Geometry: final body of the model. Coordinates: model frame, mm. Coordinates: 2 decimals unless noted, no trailing zeros. Loops run counter-clockwise (first coordinate to the right, second up) from the corner with the lowest first, then second, coordinate; pieces in that order, holes last. Notation, with made-up numbers: (17.5, 60) -> (59.5, 60) arc R24 ccw to (59.5, 81) -> close; hole circle Ø2 at (51, -26.5). An arc over 180 degrees is marked (long way). One line per item, written item: value. Start each with the question number.
Item 1: Section query B-B on x = 0. Return loops of the section in (y, z), then the cut area to 3 significant figures.
Item 2: Section query D-D on z = 28.5. Return loops of the section in (x, y), then the cut area to 3 significant figures.
Item 3: Ray query, probe 1 along Z at (x, y) = (0, 8.85); probe 2 along Z at (x, y) = (0, 7.35); probe 3 along X at (y, z) = (9, 38). Return the intervals inside material, ascending. Write a range as from..to.
Item 4: Contact query for flat-ended pins moving along their axis: pin 1 Ø1 at (x, y) = (-5.5, 7.5) entering from -Z; pin 2 Ø1 at (x, z) = (-3, 20.5) entering from -Y; pin 3 Ø4 at (x, z) = (0, 23.6) entering from -Y; pin 4 Ø2 at (y, z) = (6, 32.5) entering from -X. Output: stop coordinate, or through.
Item 5: Mould query, pull axis Y, two halves, no side actions, for faces 1 (the cylindrical face through (0.07, 9.27, 37.53)), 2 (the flat face through (0, 7, 0)), 3 (the cylindrical face through (-3.21, 9.47, 23.27)), 4 (the flat face through (8, 0, 23)). Classes: +Y half, -Y half, draft (parallel to the pull), parting line (faces both ways), or undercut.
Item 6: Section query A-A on y = 5.25. Return loops of the section in (x, z), then the cut area to 3 significant figures.
Item 7: Section query C-C on z = 23.6. Return loops of the section in (x, y), then the cut area to 3 significant figures.
from build123d import *

# Parameters (mm, degrees)
BOSS_EXTRUDE1_DEPTH     = 47.2
CUT_EXTRUDE1_DEPTH      = 50.273116402
CUT_EXTRUDE1_DEPTH_BACK = 50.273116402
SKETCH3_R               = 1.5
CUT_EXTRUDE3_DEPTH      = 51.597430898
CUT_EXTRUDE3_DEPTH_BACK = 51.597430898
SKETCH7_R               = 1.5
CUT_EXTRUDE4_DEPTH      = 37.999869057
CUT_EXTRUDE4_DEPTH_BACK = 37.999869057
SKETCH10_R              = 1.5


with BuildPart() as part:
    # Sketch1 → Boss-Extrude1 (new body)
    with BuildSketch(Plane.XY):
        with BuildLine():
            Line((6.5, 0), (10, 0))
            ThreePointArc((10, 0), (0, 10), (-10, 0))
            Line((-10, 0), (-6.5, 0))
            ThreePointArc((-6.5, 0), (0, 6.5), (6.5, 0))
        make_face()
    extrude(amount=BOSS_EXTRUDE1_DEPTH)

    # Sketch3 → Cut-Extrude1 (cut, two sides: drawn at the far end of the back side and taken through both)
    with BuildSketch(Plane(origin=(0, 0, 0), x_dir=(1, 0, 0), z_dir=(0, 1, 0)).offset(-CUT_EXTRUDE1_DEPTH_BACK)):
        with Locations(Location((0, -23.6, 0), (0, 0, 270))):
            Circle(SKETCH3_R)
    extrude(amount=CUT_EXTRUDE1_DEPTH + CUT_EXTRUDE1_DEPTH_BACK, mode=Mode.SUBTRACT)

    # Sketch7 → Cut-Extrude3 (cut, two sides: drawn at the far end of the back side and taken through both)
    with BuildSketch(Plane(origin=(0, 1.7, -1.7), x_dir=(0, 0.7071067811865389, 0.7071067811865561), z_dir=(0, 0.7071067811865561, -0.7071067811865389)).offset(-CUT_EXTRUDE3_DEPTH_BACK)):
        with Locations((11.737972568, 0)):
            Circle(SKETCH7_R)
    extrude(amount=CUT_EXTRUDE3_DEPTH + CUT_EXTRUDE3_DEPTH_BACK, mode=Mode.SUBTRACT)

    # Sketch10 → Cut-Extrude4 (cut, two sides: drawn at the far end of the back side and taken through both)
    with BuildSketch(Plane(origin=(0, 25.189187146, 25.189187146), x_dir=(0, -0.7071067811865488, 0.7071067811865464), z_dir=(0, 0.7071067811865464, 0.7071067811865488)).offset(-CUT_EXTRUDE4_DEPTH_BACK)):
        with Locations((21.480754463, 0)):
            Circle(SKETCH10_R)
    extrude(amount=CUT_EXTRUDE4_DEPTH + CUT_EXTRUDE4_DEPTH_BACK, mode=Mode.SUBTRACT)


solid = part.part
Reply:
1. outline: (6.5, 0) -> (10, 0) -> (10, 4.48) -> (6.5, 7.98) -> close; (6.5, 12.22) -> (10, 8.72) -> (10, 22.1) -> (6.5, 22.1) -> close; (6.5, 25.1) -> (10, 25.1) -> (10, 38.26) -> (6.5, 34.76) -> close; (6.5, 39) -> (10, 42.5) -> (10, 47.2) -> (6.5, 47.2) -> close
1. area: 125 mm²
2. outline: (-10, 0) -> (-6.5, 0) arc R6.5 cw to (6.5, 0) -> (10, 0) arc R10 ccw to start
2. area: 90.7 mm²
3. probe 1: z = 0..5.63, 9.87..22.1, 25.1..37.11, 41.35..47.2
3. probe 2: z = 0..7.13, 11.37..22.1, 25.1..35.61, 39.85..47.2
3. probe 3: x = -4.36..-1.14, 1.14..4.36
4. pin 1: stops at z = 0
4. pin 2: stops at y = 5.48
4. pin 3: stops at y = 6.18
4. pin 4: stops at x = -8.66
5. face 1: undercut
5. face 2: draft
5. face 3: +Y half
5. face 4: -Y half
6. outline: (-8.51, 0) -> (-3.83, 0) -> (-3.83, 47.2) -> (-8.51, 47.2) -> close; (3.83, 0) -> (8.51, 0) -> (8.51, 47.2) -> (3.83, 47.2) -> close
6. area: 442 mm²
7. outline: (-10, 0) -> (-6.5, 0) arc R6.5 cw to (-1.5, 6.32) -> (-1.5, 9.89) arc R10 ccw to start; (1.5, 6.32) arc R6.5 cw to (6.5, 0) -> (10, 0) arc R10 ccw to (1.5, 9.89) -> close
7. area: 80.2 mm²
